```python
from build123d import *

# Parameters (mm, degrees)
SKETCH1_R            = 7.6
SKETCH1_R_2          = 2
BOSS_EXTRUDE2_DEPTH  = 16
CUT_EXTRUDE1_DEPTH   = 12
SKETCH3_R            = 2
CUT_EXTRUDE2_DEPTH   = 3
SKETCH4_W            = 19.148912363
SKETCH4_H            = 4
SKETCH4_W_2          = 1.506114963
SKETCH4_H_2          = 2
SKETCH4_W_3          = 17.088400717
CUT_EXTRUDE3_DEPTH   = 34
SKETCH5_R            = 1.6
CUT_EXTRUDE4_DEPTH   = 8
SKETCH6_R            = 1.6
BOSS_EXTRUDE4_DEPTH  = 7
BOSS_EXTRUDE7_START  = -1
SKETCH9_R            = 1.6
BOSS_EXTRUDE7_DEPTH  = 1
CHAMFER2_START       = 5.004712753
CHAMFER2_DEPTH       = 3.995287247
CHAMFER2_2_DEPTH     = 5.004712753
CHAMFER2_START_2     = -28.681393589
CHAMFER2_3_OUTLINE_W = 6
CHAMFER2_3_OUTLINE_H = 10
CHAMFER2_3_DEPTH     = 3.538866325


with BuildPart() as part:
    # Sketch1 → Boss-Extrude2 (new body)
    with BuildSketch(Plane(origin=(0, 0, 0), x_dir=(1, 0, 0), z_dir=(0, 1, 0))):
        with BuildLine():
            Line((-6.773390856, -35.556903049), (7.560970701, -35.556903049))
            Line((7.560970701, -35.556903049), (17.696894961, -25.420978788))
            Line((17.696894961, -25.420978788), (23.251588719, 3.383405224))
            ThreePointArc((23.251588719, 3.383405224), (23.336919229, 3.930241848), (23.365463973, 4.482959485))
            Line((23.365463973, 4.482959485), (23.363235853, 4.637571356))
            Line((23.363235853, 4.637571356), (23.264685107, 11.476123671))
            ThreePointArc((23.264685107, 11.476123671), (21.66723092, 15.195624527), (17.911941271, 16.707029882))
            ThreePointArc((17.911941271, 16.707029882), (14.188498301, 15.136475123), (12.650070184, 11.399643748))
            Line((12.650070184, 11.399643748), (12.634536027, 4.482959485))
            ThreePointArc((12.634536027, 4.482959485), (11.321507594, 1.313028433), (8.151576542, 0))
            Line((8.151576542, 0), (7.167180778, 0))
            Line((7.167180778, 0), (0, 0))
            Line((0, 0), (-7.167180778, 0))
            Line((-7.167180778, 0), (-8.151576542, 0))
            ThreePointArc((-8.151576542, 0), (-11.321507594, 1.313028433), (-12.634536027, 4.482959485))
            Line((-12.634536027, 4.482959485), (-12.650070184, 11.399643748))
            ThreePointArc((-12.650070184, 11.399643748), (-14.188498301, 15.136475123), (-17.911941271, 16.707029882))
            ThreePointArc((-17.911941271, 16.707029882), (-21.66723092, 15.195624527), (-23.264685107, 11.476123671))
            Line((-23.264685107, 11.476123671), (-23.363235853, 4.637571356))
            Line((-23.363235853, 4.637571356), (-23.365463973, 4.482959485))
            ThreePointArc((-23.365463973, 4.482959485), (-23.336919229, 3.930241848), (-23.251588719, 3.383405224))
            Line((-23.251588719, 3.383405224), (-17.303105039, -25.027188866))
            Line((-17.303105039, -25.027188866), (-6.773390856, -35.556903049))
        make_face()
        with Locations(Location((0.196894961, -18.056903049, 0), (0, 0, 270))):
            Circle(SKETCH1_R, mode=Mode.SUBTRACT)
        with Locations(Location((-18, 4.482959485, 0), (0, 0, 270))):
            Circle(SKETCH1_R_2, mode=Mode.SUBTRACT)
        with Locations(Location((18, 4.482959485, 0), (0, 0, 270))):
            Circle(SKETCH1_R_2, mode=Mode.SUBTRACT)
    extrude(amount=BOSS_EXTRUDE2_DEPTH)

    # Sketch2 → Cut-Extrude1 (cut)
    with BuildSketch(Plane(origin=(0, 16, 0), x_dir=(1, 0, 0), z_dir=(0, 1, 0))):
        Polygon((-6.451232715, -34.106903049), (6.845022637, -34.106903049), (16.246894961, -24.705030725), (16.246894961, -11.408775373), (6.845022637, -2.006903049), (-6.451232715, -2.006903049), (-15.853105039, -11.408775373), (-15.853105039, -24.705030725), align=None)
    extrude(amount=-CUT_EXTRUDE1_DEPTH, mode=Mode.SUBTRACT)

    # Sketch3 → Cut-Extrude2 (cut)
    with BuildSketch(Plane(origin=(0, 4, 0), x_dir=(1, 0, 0), z_dir=(0, 1, 0))):
        with Locations((7.796894961, -18.056903049)):
            Circle(SKETCH3_R)
        with Locations((-7.403105039, -18.056903049)):
            Circle(SKETCH3_R)
    extrude(amount=-CUT_EXTRUDE2_DEPTH, mode=Mode.SUBTRACT)

    # Sketch4 → Cut-Extrude3 (cut)
    with BuildSketch(Plane(origin=(0, 0, 0), x_dir=(-1, 0, 0), z_dir=(0, 0, -1))):
        with Locations((17.726032724, 8)):
            Rectangle(SKETCH4_W, SKETCH4_H)
        Polygon((8.151576542, 10), (1.506114963, 10), (1.506114963, 8), (1.506114963, 6), (8.151576542, 6), align=None)
        Polygon((0, 8), (0, 10), (-8.151576542, 10), (-8.151576542, 6), (0, 6), align=None)
        with Locations((0.753057482, 9)):
            Rectangle(SKETCH4_W_2, SKETCH4_H_2)
        with Locations((0.753057482, 7)):
            Rectangle(SKETCH4_W_2, SKETCH4_H_2)
        with Locations((-16.695776901, 8)):
            Rectangle(SKETCH4_W_3, SKETCH4_H)
    extrude(amount=CUT_EXTRUDE3_DEPTH, mode=Mode.SUBTRACT)

    # Sketch5 → Cut-Extrude4 (cut)
    with BuildSketch(Plane(origin=(0, 16, 0), x_dir=(1, 0, 0), z_dir=(0, 1, 0))):
        with Locations(Location((16.246894961, -3.408775373, 0), (0, 0, 270))):
            Circle(SKETCH5_R)
        with Locations(Location((-15.853105039, -3.408775373, 0), (0, 0, 270))):
            Circle(SKETCH5_R)
    extrude(amount=-CUT_EXTRUDE4_DEPTH, mode=Mode.SUBTRACT)

    # Sketch6 → Boss-Extrude4 (add)
    with BuildSketch(Plane(origin=(0, 16, 0), x_dir=(1, 0, 0), z_dir=(0, 1, 0))):
        with BuildLine():
            Line((3.196894961, -35.556903049), (-2.803105039, -35.556903049))
            Line((-2.803105039, -35.556903049), (-2.803105039, -37.561615802))
            ThreePointArc((-2.803105039, -37.561615802), (0.196894961, -40.561615802), (3.196894961, -37.561615802))
            Line((3.196894961, -37.561615802), (3.196894961, -35.556903049))
        make_face()
        with Locations(Location((0.196894961, -37.561615802, 0), (0, 0, 270))):
            Circle(SKETCH6_R, mode=Mode.SUBTRACT)
    extrude(amount=-BOSS_EXTRUDE4_DEPTH)

    # Sketch9 → Boss-Extrude7 (add)
    with BuildSketch(Plane.XZ.offset(-9).offset(BOSS_EXTRUDE7_START)):
        with Locations(Location((0.196894961, 37.561615802, 0), (0, 0, 90))):
            Circle(SKETCH9_R)
    extrude(amount=BOSS_EXTRUDE7_DEPTH)

    # Chamfer2: read off the stored shape, not the designer's step
    # Chamfer2 outline → Chamfer2 (add)
    with BuildSketch(Plane(origin=(0, 0, 0), x_dir=(1, 0, 0), z_dir=(0, 1, 0)).offset(CHAMFER2_START)):
        with BuildLine():
            ThreePointArc((-2.803105039, -37.561615802), (0.196894961, -40.561615802), (3.196894961, -37.561615802))
            Line((3.196894961, -37.561615802), (3.196894961, -35.556903049))
            Line((3.196894961, -35.556903049), (-2.803105039, -35.556903049))
            Line((-2.803105039, -35.556903049), (-2.803105039, -37.561615802))
        make_face()
    extrude(amount=CHAMFER2_DEPTH)

    # Chamfer2 2 outline → Chamfer2 2 (add)
    with BuildSketch(Plane(origin=(0, 0, 0), x_dir=(1, 0, 0), z_dir=(0, 1, 0))):
        with BuildLine():
            ThreePointArc((-2.803105039, -37.561615802), (0.196894961, -40.561615802), (3.196894961, -37.561615802))
            Line((3.196894961, -37.561615802), (3.196894961, -35.556903049))
            Line((3.196894961, -35.556903049), (-2.803105039, -35.556903049))
            Line((-2.803105039, -35.556903049), (-2.803105039, -37.561615802))
        make_face()
    extrude(amount=CHAMFER2_2_DEPTH)

    # Chamfer2 3 outline → Chamfer2 3 (cut)
    with BuildSketch(Plane(origin=(0, 0, 0), x_dir=(1, 0, 0), z_dir=(0, 0.7071067811865511, -0.7071067811865441)).offset(CHAMFER2_START_2)):
        with Locations((0.196894961, -29)):
            Rectangle(CHAMFER2_3_OUTLINE_W, CHAMFER2_3_OUTLINE_H)
    extrude(amount=CHAMFER2_3_DEPTH, mode=Mode.SUBTRACT)


solid = part.part
```
Can you work these out from the model? Positions are in its coordinate system, mm. A direction names the side the tool comes from. Coordinates: 2 decimals unless noted, no trailing zeros. Loops run counter-clockwise (first coordinate to the right, second up) from the corner with the lowest first, then second, coordinate; pieces in that order, holes last.
Item 1: Suppose I cut it at A-A (z = 22.5). Please give me the cut outline in (x, y), then the cut area to 3 significant figures.
Answers below:
outline: (-17.83, 0) - (-5.97, 0) - (-5.97, 4) - (-15.85, 4) - (-15.85, 16) - (-17.83, 16) - close; (6.36, 0) - (18.26, 0) - (18.26, 16) - (16.25, 16) - (16.25, 4) - (6.36, 4) - close
area: 143 mm2
Item 2: If we mould it in two halves opening along Z, with no side actions, what happens to faces 4 (the face through (17, 10, -8)), 5 (the face through (9.796, 2.521, 18.105))? For each: released by +Z, released by -Z, zero draft, split by the parting line, or undercut.
Answers below:
face 4: zero draft
face 5: undercut
Item 3: Please list where these lines run through material, in increasing order: L1, parallel to Y at x = -13, z = -10; L2, parallel to Z at x = 15.5, y = 8.5; L3, parallel to Z at x = 3.5, y = 9.5.
Answers below:
L1: y = 0 to 6, 10 to 16
L2: z = 0 to 1.99, 4.82 to 10.66, 25.45 to 27.62
L3: z = 0 to 2.01, 34.11 to 35.56
Item 4: Which directions (+Z, -Z, +X, -X, +Y, -Y) give clear straight access to the entire face, cutting with the end or side of a thin tool? Please do faces 1 (the face through (0, 0, 9)), 2 (the face through (18, 6, -8)), 3 (the face through (-15.853, 10, 18)).
Answers below:
face 1: +Z, -Z, +X, -X, -Y
face 2: -Z, +X, -X
face 3: +Y
Item 5: Suppose I cut it at D-D (y = 13.5). State how many separate pieces and enclosed holes the cut face has, then the cut area to 3 significant figures.
Answers below:
separate pieces: 1
enclosed holes: 6
area: 727 mm2
Item 6: I'm going to push flat-ended pins straight in: pin 1 (6 mm diameter, centred on y = 10, z = 15.5, fed in from -X); pin 2 (16 mm diameter, centred on x = 2.5, z = 25.5, fed in from +Y); pin 3 (5 mm diameter, centred on x = -11.5, y = 2.5, fed in from -Z). Where does each tip first touch, or does it pass through?
Answers below:
pin 1: stops at x = -19.93
pin 2: stops at y = 4
pin 3: stops at z = -14.94
Item 7: Suppose I cut it at C-C (z = 9). Please give me the cut outline in (x, y).
Answers below:
outline: (-20.66, 0) - (20.86, 0) - (20.86, 16) - (13.84, 16) - (13.84, 4) - (-13.44, 4) - (-13.44, 16) - (-20.66, 16) - close
Item 8: Suppose I cut it at B-B (x = 4.5). Please give me the cut outline in (y, z).
Answers below:
outline: (0, 0) - (16, 0) - (16, 2.01) - (4, 2.01) - (4, 11.79) - (0, 11.79) - close; (0, 24.32) - (4, 24.32) - (4, 34.11) - (16, 34.11) - (16, 35.56) - (0, 35.56) - close
